```python
from build123d import *

# Parameters (mm, degrees)
CROQUIS1_R              = 1.75
CROQUIS1_R_2            = 1.65
SALIENTE_EXTRUIR1_DEPTH = 59.54
CROQUIS2_W              = 3.035
CROQUIS2_H              = 7
CROQUIS2_W_2            = 6.07
CORTAR_EXTRUIR1_DEPTH   = 149.131714596


with BuildPart() as part:
    # Croquis1 → Saliente-Extruir1 (new body)
    with BuildSketch(Plane.XY):
        with BuildLine():
            Line((-13.171572875, -18.828427125), (2.828427125, -2.828427125))
            ThreePointArc((2.828427125, -2.828427125), (3.69551813, -1.530733729), (4, 0))
            Line((4, 0), (4, 129.999038458))
            ThreePointArc((4, 129.999038458), (0.513461538, 133.49901257), (-2.99989645, 130.025961336))
            Line((-2.99989645, 130.025961336), (-3.987275146, 1.669579104))
            Line((-3.987275146, 1.669579104), (-18.828427125, -13.171572875))
            ThreePointArc((-18.828427125, -13.171572875), (-18.828427125, -18.828427125), (-13.171572875, -18.828427125))
        make_face()
        Circle(CROQUIS1_R, mode=Mode.SUBTRACT)
        with Locations((-16, -16)):
            Circle(CROQUIS1_R, mode=Mode.SUBTRACT)
        with Locations((0.5, 129.999038458)):
            Circle(CROQUIS1_R_2, mode=Mode.SUBTRACT)
    extrude(amount=-SALIENTE_EXTRUIR1_DEPTH)

    # Croquis2 → Cortar-Extruir1 (cut, through all)
    with BuildSketch(Plane(origin=(4, 0, 0), x_dir=(0, 0, -1), z_dir=(1, 0, 0))):
        Polygon((2, 4), (2, -20), (57.54, -20), (57.54, 4), (55.54, 4), (4, 4), align=None)
        with Locations((28.2525, 129.999038458)):
            Rectangle(CROQUIS2_W, CROQUIS2_H)
        with Locations((31.2875, 129.999038458)):
            Rectangle(CROQUIS2_W, CROQUIS2_H)
        Polygon((4, 34), (4, 4), (55.54, 4), (55.54, 34), (29.77, 34), align=None)
        Polygon((17.984568448, 121.580171608), (4, 34), (29.77, 34), (29.77, 121.580171608), align=None)
        Polygon((29.77, 34), (55.54, 34), (41.555431552, 121.580171608), (29.77, 121.580171608), align=None)
        Polygon((14.77, 126.499038458), (14.77, 133.499038458), (0, 133.499038458), (0, 34), align=None)
        with Locations((17.805, 129.999038458)):
            Rectangle(CROQUIS2_W_2, CROQUIS2_H)
        Polygon((44.77, 126.499038458), (59.54, 34), (59.54, 133.499038458), (44.77, 133.499038458), align=None)
        with Locations((41.735, 129.999038458)):
            Rectangle(CROQUIS2_W_2, CROQUIS2_H)
    extrude(amount=-CORTAR_EXTRUIR1_DEPTH, mode=Mode.SUBTRACT)


solid = part.part
```
The listing builds one solid part. Answer for the finished solid, in the listing's coordinates (mm). A direction names the side the tool comes from. Round coordinates to 2 decimals unless told otherwise and drop trailing zeros. Order: outer loops, then holes, each group sorted by start corner. A loop starts at its lowest first (then second) coordinate and runs counter-clockwise, first axis right, second up. Notation, with made-up numbers: (68, 70) -> (111, 70) arc R28 cw to (111, 101) -> close; hole circle Ø8 at (88, 24). An arc over 180 degrees is marked (long way). Answer as CSV lines item,"result". Start each with the question number.
(1) A tool of negligible diameter and unlimited length cuts with its end or side. For faces 1 (the face through (1, 128, -38.7)), 2 (the face through (0.18, 78.4, -11.09)), 3 (the face through (1, 128, -32.805)), 4 (the face through (1, 126.499, -18)), from which of +Z, -Z, +X, -X, +Y, -Y can it reach the whole face along a straight path? Write none if from no direction.
(2) The part is cut by section A-A (y = 106.5). Determine the outline of the cut face in (x, z), then the cut area to 3 significant figures.
(3) Find the intervals of material crossed by probe 1 along Z at (x, y) = (1, 14); probe 2 along Z at (x, y) = (-8, -11.5); probe 3 along Y at (x, z) = (-16, -58.05), in increasing order. Write a range as from..to.
(4) The part is cut by section B-B (x = -16). Determine the outline of the cut face in (y, z).
(5) For a pull along X with two mould halves and no side action, classify faces 5 (the face through (-11.304, -5.647, -58.526)), 6 (the face through (0.18, 79.6, -7.28)), 7 (the face through (1.617, -0.67, -0.986)) as +X half, -X half, draft (parallel to the pull), parting line (faces both ways), or undercut.
(6) The part is cut by section C-C (x = -8). Determine the outline of the cut face in (y, z).
(7) Flat-ended cylindrical pins translate along their axes: pin 1 Ø3 at (x, z) = (0, -18) entering from +Y; pin 2 Ø3.5 at (x, y) = (1.5, 130) entering from +Z; pin 3 Ø7.5 at (x, y) = (2, 128.5) entering from -Z; pin 4 Ø2.5 at (x, y) = (0, 18) entering from +Z. Find the tip coordinate at first contact, or state that the pin passes through.
Evaluation:
1,face 1,"-Z, +X, -X, +Y"
1,face 2,"+X, -X, -Y"
1,face 3,"+X, -X, +Y"
1,face 4,"+Z, +X, -X, +Y"
2,outline,"(-3.18, -47.96) -> (4, -47.96) -> (4, -43.96) -> (-3.18, -43.96) -> close; (-3.18, -15.58) -> (4, -15.58) -> (4, -11.58) -> (-3.18, -11.58) -> close"
2,area,"57.4 mm²"
3,probe 1,"-59.54..-55.54, -4..0"
3,probe 2,"-59.54..-57.54, -2..0"
3,probe 3,"-20..-17.75, -14.25..-10.34"
4,outline,"(-20, -59.54) -> (-17.75, -59.54) -> (-17.75, -57.54) -> (-20, -57.54) -> close; (-20, -2) -> (-17.75, -2) -> (-17.75, 0) -> (-20, 0) -> close; (-14.25, -59.54) -> (-10.34, -59.54) -> (-10.34, -57.54) -> (-14.25, -57.54) -> close; (-14.25, -2) -> (-10.34, -2) -> (-10.34, 0) -> (-14.25, 0) -> close"
5,face 5,"-X half"
5,face 6,"draft"
5,face 7,"undercut"
6,outline,"(-13.66, -59.54) -> (-2.34, -59.54) -> (-2.34, -57.54) -> (-13.66, -57.54) -> close; (-13.66, -2) -> (-2.34, -2) -> (-2.34, 0) -> (-13.66, 0) -> close"
7,pin 1,"y = 126.5"
7,pin 2,"z = -20.84"
7,pin 3,"z = -45.05"
7,pin 4,"z = 0"
